```python
from build123d import *

# Parameters (mm, degrees)
F0_W     = 115
F0_H     = 115
F1_DEPTH = 10
F2_W     = 83
F2_H     = 62
F3_DEPTH = 6
F4_W     = 1
F4_H     = 62
F5_DEPTH = 6
F7_DEPTH = 8


# Not quite as in the source:
# - a feature of the source that left no trace in its solid (it failed there, or was rolled back) is left out


with BuildPart() as f1:
    # F0 (on Top) → F1 (new body)
    with BuildSketch(Plane.XY):
        Rectangle(F0_W, F0_H)
    extrude(amount=F1_DEPTH)

    # F2 (on face) → F3 (cut)
    with BuildSketch(Plane(origin=(0, 0, 0), x_dir=(1, 0, 0), z_dir=(0, 0, -1))):
        Rectangle(F2_W, F2_H)
    extrude(amount=-F3_DEPTH, mode=Mode.SUBTRACT)

    # F4 (on face) → F5 (join)
    with BuildSketch(Plane(origin=(0, 0, 0), x_dir=(1, 0, 0), z_dir=(0, 0, -1))):
        Rectangle(F4_W, F4_H)
    extrude(amount=-F5_DEPTH)

    # F6 (on face) → F7 (cut)
    with BuildSketch(Plane(origin=(0, 0, 0), x_dir=(1, 0, 0), z_dir=(0, 0, -1))):
        Polygon((-39.3114286867, 50.5), (-55.8729671482, 50.5), (-41.8729671482, 32), align=None)
        Polygon((-56.5, 33.1098824129), (-42.5, 31.1714208744), (-56.5, 49.6714208744), align=None)
        Polygon((-38.3018883964, 50.5), (-40.863426858, 32), (-24.3018883964, 32), align=None)
        Polygon((-20.4862842313, 50.5), (-37.0478226928, 50.5), (-23.0478226928, 32), align=None)
        Polygon((-19.4767439411, 50.5), (-22.0382824026, 32), (-5.4767439411, 32), align=None)
        Polygon((-1.0149211209, 50.5), (-18.2226782375, 50.5), (-4.2226782375, 32), align=None)
        Polygon((0, 50.5), (-3.2050376771, 32.0156837407), (3.2131379472, 32), align=None)
        Polygon((4.2226782375, 32), (18.2226782375, 50.5), (1.0149211209, 50.5), align=None)
        Polygon((22.0382824026, 32), (19.4767439411, 50.5), (5.4767439411, 32), align=None)
        Polygon((20.4862842313, 50.5), (23.0478226928, 32), (37.0478226928, 50.5), align=None)
        Polygon((40.863426858, 32), (38.3018883964, 50.5), (24.3018883964, 32), align=None)
        Polygon((39.3114286867, 50.5), (41.8729671482, 32), (55.8729671482, 50.5), align=None)
        Polygon((56.5, 49.6714208744), (42.5, 31.1714208744), (56.5, 33.1098824129), align=None)
        Polygon((-42.5, 13.6003421226), (-42.5, 30.1618805842), (-56.5, 32.1003421226), align=None)
        Polygon((-42.5, 11.9431838715), (-56.5, 30.4431838715), (-56.5, 13.8816454099), align=None)
        Polygon((-42.5, 1.2975080085), (-42.5, 10.9336435812), (-56.5, 12.8721051197), align=None)
        Polygon((-56.5, -13.8816454099), (-56.5, -30.4431838715), (-42.5, -11.9431838715), align=None)
        Polygon((-42.5, -13.6003421226), (-56.5, -32.1003421226), (-42.5, -30.1618805842), align=None)
        Polygon((-56.5, -49.6714208744), (-42.5, -31.1714208744), (-56.5, -33.1098824129), align=None)
        Polygon((-41.8729671482, -32), (-55.8729671482, -50.5), (-39.3114286867, -50.5), align=None)
        Polygon((56.5, 32.1003421226), (42.5, 30.1618805842), (42.5, 13.6003421226), align=None)
        Polygon((42.5, 11.9431838715), (56.5, 13.8816454099), (56.5, 30.4431838715), align=None)
        Polygon((56.5, -13.8816454099), (42.5, -11.9431838715), (56.5, -30.4431838715), align=None)
        Polygon((42.5, -30.1618805842), (56.5, -32.1003421226), (42.5, -13.6003421226), align=None)
        Polygon((56.5, -33.1098824129), (42.5, -31.1714208744), (56.5, -49.6714208744), align=None)
        Polygon((39.3114286867, -50.5), (55.8729671482, -50.5), (41.8729671482, -32), align=None)
        Polygon((-38.3018883964, -50.5), (-24.3018883964, -32), (-40.863426858, -32), align=None)
        Polygon((-23.0478226928, -32), (-37.0478226928, -50.5), (-20.4862842313, -50.5), align=None)
        Polygon((-5.4767439411, -32), (-22.0382824026, -32), (-19.4767439411, -50.5), align=None)
        Polygon((-4.2226782375, -32), (-18.2226782375, -50.5), (-1.0149211209, -50.5), align=None)
        Polygon((1.0149211209, -50.5), (18.2226782375, -50.5), (4.2226782375, -32), align=None)
        Polygon((5.4767439411, -32), (19.4767439411, -50.5), (22.0382824026, -32), align=None)
        Polygon((37.0478226928, -50.5), (23.0478226928, -32), (20.4862842313, -50.5), align=None)
        Polygon((24.3018883964, -32), (38.3018883964, -50.5), (40.863426858, -32), align=None)
        Polygon((3.2131379472, -32), (-3.2050376771, -32.0156837407), (0, -50.5), align=None)
        Polygon((56.5, 12.8721051197), (42.5, 10.9336435812), (42.5, 1.2975080085), align=None)
        Polygon((-42.5, 0), (-56.5, 11.5745971112), (-56.5, -11.5745971112), align=None)
        Polygon((56.5, -11.5745971112), (56.5, 11.5745971112), (42.5, 0), align=None)
        Polygon((-42.5, -10.9431838715), (-42.5, -1.2975080085), (-56.5, -12.8721051197), align=None)
        Polygon((42.5, -10.9431838715), (56.5, -12.8721051197), (42.5, -1.2975080085), align=None)
    extrude(amount=-F7_DEPTH, mode=Mode.SUBTRACT)


solid = f1.part
```
Could you check a few things on this model? Use its own coordinates, in mm. Give positions to 0.01 mm unless a question says otherwise; leave off trailing zeros. Loops run counter-clockwise (first coordinate to the right, second up) from the corner with the lowest first, then second, coordinate; pieces in that order, holes last. Notation, with made-up numbers: (5, 85) - (33, 85) arc R13 cw to (33, 101) - close; hole circle Ø9 at (20, 26). An arc over 180 degrees is marked (long way). Use one line per item in the form item = value.
1. I want a section at A-A (z = 3). Give the number of separate pieces and of enclosed holes in the cut face, and give its area (3 significant figures).
Response values:
separate_pieces = 1
enclosed_holes = 42
area = 2,950 mm²
2. I want a section at C-C (x = 28). Please give me the cut outline in (y, z).
Response values:
outline = (-57.5, 0) - (-50.5, 0) - (-50.5, 8) - (-38.54, 8) - (-38.54, 0) - (-36.89, 0) - (-36.89, 8) - (-32, 8) - (-32, 0) - (-31, 0) - (-31, 6) - (31, 6) - (31, 0) - (32, 0) - (32, 8) - (36.89, 8) - (36.89, 0) - (38.54, 0) - (38.54, 8) - (50.5, 8) - (50.5, 0) - (57.5, 0) - (57.5, 10) - (-57.5, 10) - close
3. I want a section at D-D (y = -23). Please give me the cut outline in (x, z), and give its area (3 significant figures).
Response values:
outline = (-57.5, 0) - (-56.5, 0) - (-56.5, 8) - (-50.87, 8) - (-50.87, 0) - (-49.61, 0) - (-49.61, 8) - (-42.5, 8) - (-42.5, 0) - (-41.5, 0) - (-41.5, 6) - (-0.5, 6) - (-0.5, 0) - (0.5, 0) - (0.5, 6) - (41.5, 6) - (41.5, 0) - (42.5, 0) - (42.5, 8) - (49.61, 8) - (49.61, 0) - (50.87, 0) - (50.87, 8) - (56.5, 8) - (56.5, 0) - (57.5, 0) - (57.5, 10) - (-57.5, 10) - close
area = 454 mm²
4. I want a section at B-B (y = -3.5). Please give me the cut outline in (x, z).
Response values:
outline = (-57.5, 0) - (-56.5, 0) - (-56.5, 8) - (-46.73, 8) - (-46.73, 0) - (-45.16, 0) - (-45.16, 8) - (-42.5, 8) - (-42.5, 0) - (-41.5, 0) - (-41.5, 6) - (-0.5, 6) - (-0.5, 0) - (0.5, 0) - (0.5, 6) - (41.5, 6) - (41.5, 0) - (42.5, 0) - (42.5, 8) - (45.16, 8) - (45.16, 0) - (46.73, 0) - (46.73, 8) - (56.5, 8) - (56.5, 0) - (57.5, 0) - (57.5, 10) - (-57.5, 10) - close
5. I need wall thicknesses on probe 1 along Y at (x, z) = (-33, 7.5); probe 2 along Y at (x, z) = (-33, 4.75); probe 3 along X at (y, z) = (-24.5, 6.25). Which ranges of each line are inside material? Lowest first, please.
Response values:
probe_1 = -57.5 to -50.5, -45.15 to -43.49, -32 to 32, 43.49 to 45.15, 50.5 to 57.5
probe_2 = -57.5 to -50.5, -45.15 to -43.49, -32 to -31, 31 to 32, 43.49 to 45.15, 50.5 to 57.5
probe_3 = -57.5 to -56.5, -52 to -50.75, -42.5 to 42.5, 50.75 to 52, 56.5 to 57.5
6. I'm going to push flat-ended pins straight in: pin 1 Ø4 at (x, y) = (-51, 37) entering from -Z; pin 2 Ø2 at (x, y) = (-17.5, 18.5) entering from -Z. Where does each tip first touch, or does it pass through?
Response values:
pin_1 = 8
pin_2 = 6
